Read the model definition and answer for the solid it produces. Units are mm, in the model's axes. A direction names the side the tool comes from. Coordinates: 2 decimals unless noted, no trailing zeros. Write each loop counter-clockwise with the first axis right and the second up, starting at its lowest first coordinate (ties: lowest second). Pieces come first, ordered by that corner, then holes.
Item 1: Straight lines are drawn through the part: probe 1 along Y at (x, z) = (0, -23.3); probe 2 along X at (y, z) = (12.5, 20); probe 3 along X at (y, z) = (6.5, -23.85). For each, find the intervals that lie inside material, in ascending order.
Item 2: Determine the mould class of faces 6 (the face through (0, 4, -27.35)), 7 (the face through (24.5, -3, 1.5)) for opening direction X: released by +X, released by -X, zero draft, split by the parting line, or undercut.
Item 3: Section A-A (y = 1.25) is taken. State how many separate pieces and enclosed holes the cut face has, then the cut area to 3 significant figures.
Item 4: Section B-B (z = -13) is taken. Give the vertices of the cut face in (x, y).
Item 5: Each of these flat-tipped pins is pushed along its axis until it touches: P1, Ø5.5, axis at x = 16, z = -13, coming from the -Y side; P2, Ø1, axis at y = 1.5, z = -0.5, coming from the +X side; P3, Ø3.5, axis at y = 18, z = -0.5, coming from the +X side. Where does it stop, or does it pass through?
Item 6: A tool of negligible diameter and unlimited length cuts with its end or side. For faces 1 (the face through (0.37, 8.16, -32.24)), 2 (the face through (-2.901, 4, -26)), 3 (the face through (-24.43, 10.35, 20.67)), 4 (the face through (-9.57, 15.577, 2.524)), 5 (the face through (2.5, 6, -34)), from which of +Z, -Z, +X, -X, +Y, -Y can it reach the whole face along a straight path? Write none if from no direction.
Item 7: Section C-C (z = 18) is taken. Give the vertices of the cut face in (x, y), then the cut area to 3 significant figures.
from build123d import *
from build123d.topology import SkipClean

# Parameters (mm, degrees)
CORTAR_EXTRUIR1_DEPTH      = 13
CROQUIS3_R                 = 1.7
CORTAR_EXTRUIR2_DEPTH      = 17
CORTAR_EXTRUIR3_DEPTH      = 1.5
CORTAR_EXTRUIR3_DEPTH_BACK = 1.5
CROQUIS5_R                 = 5
CORTAR_EXTRUIR4_DEPTH      = 21
CROQUIS6_R                 = 8.2
CORTAR_EXTRUIR5_DEPTH      = 9
CROQUIS7_W                 = 30.6
CROQUIS7_H                 = 7
CORTAR_EXTRUIR6_DEPTH      = 4
CROQUIS8_R                 = 1.7
CORTAR_EXTRUIR7_DEPTH      = 17
CORTAR_EXTRUIR8_DEPTH      = 11
CORTAR_EXTRUIR9_DEPTH      = 21
CROQUIS11_R                = 1.7
CORTAR_EXTRUIR10_DEPTH     = 21
CROQUIS12_R                = 2.95
CORTAR_EXTRUIR11_DEPTH     = 3
BOSS_EXTRUDE1_START        = 3
SKETCH1_R                  = 7
BOSS_EXTRUDE1_DEPTH        = 3
SKETCH2_R                  = 1.7
CUT_EXTRUDE1_DEPTH         = 62.449166022
CUT_EXTRUDE2_DEPTH         = 22.5


with BuildPart() as part:
    # Croquis1 → Revolución1 (revolve)
    with BuildSketch(Plane.XY, mode=Mode.PRIVATE) as revoluci_n1_sk:
        Polygon((0, 0), (40, 0), (40, 3), (37, 3), (37, 21), (0, 21), align=None)
    revolve(revoluci_n1_sk.sketch.rotate(Axis((0, 21, 0), (0, -1, 0)), 90), axis=Axis((0, 21, 0), (0, -1, 0)))

    # Croquis2 → Cortar-Extruir1 (cut)
    with BuildSketch(Plane.XZ):
        Polygon((-11.5, -19.5), (11.5, -19.5), (11.5, -23), (5, -29.5), (5, -54.5), (2.5, -54.5), (2.5, -29.5), (9, -23), (-9, -23), (-2.5, -29.5), (-2.5, -54.5), (-5, -54.5), (-5, -29.5), (-11.5, -23), align=None)
    extrude(amount=-CORTAR_EXTRUIR1_DEPTH, mode=Mode.SUBTRACT)

    # Croquis3 → Cortar-Extruir2 (cut)
    with BuildSketch(Plane.XY.offset(-40)):
        with Locations(Location((0, 6.5, 0), (0, 0, 180))):
            Circle(CROQUIS3_R)
    extrude(amount=CORTAR_EXTRUIR2_DEPTH, mode=Mode.SUBTRACT)

    # Croquis4 → Cortar-Extruir3 (cut, two sides: drawn at the far end of the back side and taken through both)
    with BuildSketch(Plane.XY.offset(-25.85).offset(-CORTAR_EXTRUIR3_DEPTH_BACK)):
        Polygon((0, 9.85), (-2.901185103, 8.175), (-2.901185103, 4.825), (-2.901185103, -1.825), (2.901185103, -1.825), (2.901185103, 4.825), (2.901185103, 8.175), align=None)
    extrude(amount=CORTAR_EXTRUIR3_DEPTH + CORTAR_EXTRUIR3_DEPTH_BACK, mode=Mode.SUBTRACT)

    # Croquis5 → Cortar-Extruir4 (cut)
    with BuildSketch(Plane(origin=(0, 21, 0), x_dir=(1, 0, 0), z_dir=(0, 1, 0))):
        with Locations(Location((0, 0, 0), (0, 0, 270))):
            Circle(CROQUIS5_R)
    extrude(amount=-CORTAR_EXTRUIR4_DEPTH, mode=Mode.SUBTRACT)

    # Croquis6 → Cortar-Extruir5 (cut)
    with BuildSketch(Plane.XZ):
        with Locations(Location((0, 0, 0), (0, 0, 270))):
            Circle(CROQUIS6_R)
    extrude(amount=-CORTAR_EXTRUIR5_DEPTH, mode=Mode.SUBTRACT)

    # Croquis7 → Cortar-Extruir6 (cut)
    with BuildSketch(Plane.XZ):
        Rectangle(CROQUIS7_W, CROQUIS7_H)
    extrude(amount=-CORTAR_EXTRUIR6_DEPTH, mode=Mode.SUBTRACT)

    # Croquis8 → Cortar-Extruir7 (cut)
    with BuildSketch(Plane.XZ.offset(-4)):
        with Locations(Location((-11, 0, 0), (0, 0, 270))):
            Circle(CROQUIS8_R)
        with Locations(Location((11, 0, 0), (0, 0, 270))):
            Circle(CROQUIS8_R)
    extrude(amount=-CORTAR_EXTRUIR7_DEPTH, mode=Mode.SUBTRACT)

    # Croquis9 → Cortar-Extruir8 (cut)
    with BuildSketch(Plane(origin=(0, 21, 0), x_dir=(1, 0, 0), z_dir=(0, 1, 0))):
        Polygon((-11, 3.35), (-13.901185103, 1.675), (-13.901185103, -1.675), (-11, -3.35), (-8.098814897, -1.675), (-8.098814897, 1.675), align=None)
        Polygon((11, 3.35), (8.098814897, 1.675), (8.098814897, -1.675), (11, -3.35), (13.901185103, -1.675), (13.901185103, 1.675), align=None)
        Polygon((-25.916185103, 1.675), (-23.015, 3.35), (-20.113814897, 1.675), (-20.113814897, -1.675), (-23.015, -3.35), (-25.916185103, -1.675), align=None)
        Polygon((20.113814897, 1.675), (23.015, 3.35), (25.916185103, 1.675), (25.916185103, -1.675), (23.015, -3.35), (20.113814897, -1.675), align=None)
    extrude(amount=-CORTAR_EXTRUIR8_DEPTH, mode=Mode.SUBTRACT)

    # Croquis10 → Cortar-Extruir9 (cut)
    with BuildSketch(Plane.XZ):
        with BuildLine():
            Line((9.447221814, 16.363068172), (14.966629547, 25.922962794))
            ThreePointArc((14.966629547, 25.922962794), (16.245761141, 26.871003909), (17.811925712, 26.584493647))
            ThreePointArc((17.811925712, 26.584493647), (24.51342218, 20.56920351), (29.273623894, 12.924973661))
            ThreePointArc((29.273623894, 12.924973661), (29.283819798, 11.332850665), (28.128062687, 10.237777566))
            Line((28.128062687, 10.237777566), (17.754969251, 6.462280318))
            ThreePointArc((17.754969251, 6.462280318), (16.322400804, 6.487021228), (15.273989073, 7.4635955))
            ThreePointArc((15.273989073, 7.4635955), (13.022755533, 10.927389365), (10.002507082, 13.745903101))
            ThreePointArc((10.002507082, 13.745903101), (9.222823954, 14.947967445), (9.447221814, 16.363068172))
        make_face()
    cortar_extruir9 = extrude(amount=-CORTAR_EXTRUIR9_DEPTH, mode=Mode.SUBTRACT)

    # Simetría1: Cortar-Extruir9 across plane
    add(cortar_extruir9.mirror(Plane(origin=(0, 0, 0), x_dir=(0, 0, 1), z_dir=(1, 0, 0))), mode=Mode.SUBTRACT)

    # Croquis11 → Cortar-Extruir10 (cut)
    with BuildSketch(Plane.XZ):
        with Locations(Location((-16, -13, 0), (0, 0, 270))):
            Circle(CROQUIS11_R)
        with Locations(Location((16, -13, 0), (0, 0, 270))):
            Circle(CROQUIS11_R)
        with Locations(Location((0, 18, 0), (0, 0, 270))):
            Circle(CROQUIS11_R)
    extrude(amount=-CORTAR_EXTRUIR10_DEPTH, mode=Mode.SUBTRACT)

    # Croquis12 → Cortar-Extruir11 (cut)
    with BuildSketch(Plane.XZ):
        with Locations(Location((-16, -13, 0), (0, 0, 270))):
            Circle(CROQUIS12_R)
        with Locations(Location((16, -13, 0), (0, 0, 270))):
            Circle(CROQUIS12_R)
        with Locations(Location((0, 18, 0), (0, 0, 270))):
            Circle(CROQUIS12_R)
    extrude(amount=-CORTAR_EXTRUIR11_DEPTH, mode=Mode.SUBTRACT)

    # Sketch1 → Boss-Extrude1 (add)
    with SkipClean():  # the faces are left unmerged after this step: merging them gives an invalid solid
        with BuildSketch(Plane.XZ.offset(BOSS_EXTRUDE1_START)):
            with BuildLine():
                Line((-13.206887408, 7.625), (-8.660254038, 5))
                ThreePointArc((-8.660254038, 5), (0, 10), (8.660254038, 5))
                Line((8.660254038, 5), (13.206887408, 7.625))
                ThreePointArc((13.206887408, 7.625), (8.046591752, 12.954337543), (0.982257886, 15.218333333))
                ThreePointArc((0.982257886, 15.218333333), (0, 15.05), (-0.982257886, 15.218333333))
                ThreePointArc((-0.982257886, 15.218333333), (-8.046591752, 12.954337543), (-13.206887408, 7.625))
            make_face()
            with BuildLine():
                Line((13.206887408, -7.625), (8.660254038, -5))
                ThreePointArc((8.660254038, -5), (0, -10), (-8.660254038, -5))
                Line((-8.660254038, -5), (-13.206887408, -7.625))
                ThreePointArc((-13.206887408, -7.625), (0, -15.25), (13.206887408, -7.625))
            make_face()
            with Locations(Location((23.015, 0, 0), (0, 0, 90))):
                Circle(SKETCH1_R)
            with Locations(Location((-23.015, 0, 0), (0, 0, 90))):
                Circle(SKETCH1_R)
        extrude(amount=-BOSS_EXTRUDE1_DEPTH)

    # Sketch2 → Cut-Extrude1 (cut, through all)
    with SkipClean():  # the faces are left unmerged after this step: merging them gives an invalid solid
        with BuildSketch(Plane(origin=(0, -3, 0), x_dir=(-1, 0, 0), z_dir=(0, -1, 0))):
            with Locations(Location((23.015, 0, 0), (0, 0, 90))):
                Circle(SKETCH2_R)
            with Locations(Location((-23.015, 0, 0), (0, 0, 90))):
                Circle(SKETCH2_R)
        extrude(amount=-CUT_EXTRUDE1_DEPTH, mode=Mode.SUBTRACT)

    # Sketch3 → Cut-Extrude2 (cut)
    with SkipClean():  # the faces are left unmerged after this step: merging them gives an invalid solid
        with BuildSketch(Plane(origin=(0, 21, 0), x_dir=(1, 0, 0), z_dir=(0, 1, 0))):
            Polygon((-25.916185103, 1.675), (-23.015, 3.35), (-20.113814897, 1.675), (-20.113814897, -1.675), (-23.015, -3.35), (-25.916185103, -1.675), align=None)
            Polygon((23.015, 3.35), (20.113814897, 1.675), (20.113814897, -1.675), (23.015, -3.35), (25.916185103, -1.675), (25.916185103, 1.675), align=None)
        extrude(amount=-CUT_EXTRUDE2_DEPTH, mode=Mode.SUBTRACT)


solid = part.part
Established:
1. probe 1: y = 0 to 4.8, 8.2 to 21
1. probe 2: x = -31.13 to -24.98, -11.55 to 11.55, 24.98 to 31.13
1. probe 3: x = -28.29 to -10.65, -8.15 to -1.7, 1.7 to 8.15, 10.65 to 28.29
2. face 6: undercut
2. face 7: zero draft
3. separate pieces: 2
3. enclosed holes: 9
3. area: 3,880 mm2
4. outline: (-37.83, 0) - (-18.95, 0) - (-18.95, 3) - (-17.7, 3) - (-17.7, 21) - (-34.64, 21) - (-34.64, 3) - (-37.83, 3) - close; (-14.3, 3) - (-13.05, 3) - (-13.05, 0) - (-7.97, 0) - (-7.97, -3) - (7.97, -3) - (7.97, 0) - (13.05, 0) - (13.05, 3) - (14.3, 3) - (14.3, 21) - (-14.3, 21) - close; (17.7, 3) - (18.95, 3) - (18.95, 0) - (37.83, 0) - (37.83, 3) - (34.64, 3) - (34.64, 21) - (17.7, 21) - close
5. P1: stops at y = 3
5. P2: stops at x = 40
5. P3: stops at x = 37
6. face 1: -Z
6. face 2: -Y
6. face 3: +Y, -Y
6. face 4: +Y
6. face 5: -Z, -Y
7. outline: (-35.72, 0) - (-26.46, 0) - (-26.46, 21) - (-32.33, 21) - (-32.33, 3) - (-35.72, 3) - close; (-10.39, 0) - (-2.95, 0) - (-2.95, 3) - (-1.7, 3) - (-1.7, 21) - (-10.39, 21) - close; (1.7, 3) - (2.95, 3) - (2.95, 0) - (10.39, 0) - (10.39, 21) - (1.7, 21) - close; (26.46, 0) - (35.72, 0) - (35.72, 3) - (32.33, 3) - (32.33, 21) - (26.46, 21) - close
7. area: 624 mm2
